Work out the finished part from the listing and answer in its coordinate system (mm). Round coordinates to 2 decimals unless told otherwise and drop trailing zeros. Loops run counter-clockwise (first coordinate to the right, second up) from the corner with the lowest first, then second, coordinate; pieces in that order, holes last.
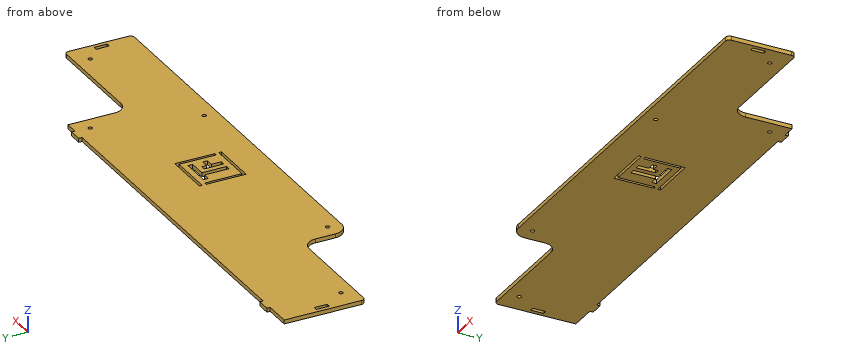
from build123d import *

# Parameters (mm, degrees)
SKETCH001002018_R = 1.5
SKETCH001002018_W = 9.8
SKETCH001002018_H = 3
PAD020_DEPTH      = 3
FILLET031_R       = 3
FILLET032_R       = 10


with BuildPart() as part:
    # Sketch001002018 → Pad020 (new body)
    with BuildSketch(Plane(origin=(0, 45, 17.5), x_dir=(0, -1, 0), z_dir=(0, 0, 1))):
        Polygon((-61, -198.5), (0, -198.5), (0, -108.5), (35, -108.5), (35, 198.5), (-16, 198.5), (-16, 108.5), (-61, 108.5), (-61, 98.5), (-63.5, 98.5), (-63.5, 88.5), (-61, 88.5), (-61, -168.5), (-63.5, -168.5), (-63.5, -178.5), (-61, -178.5), align=None)
        with Locations((-50.1, 97.5)):
            Circle(SKETCH001002018_R, mode=Mode.SUBTRACT)
        with Locations((-5.1, 182.5)):
            Circle(SKETCH001002018_R, mode=Mode.SUBTRACT)
        with Locations((24.9, 77.5)):
            Circle(SKETCH001002018_R, mode=Mode.SUBTRACT)
        with Locations((-10.1, -182.5)):
            Circle(SKETCH001002018_R, mode=Mode.SUBTRACT)
        with Locations((24.9, -97.5)):
            Circle(SKETCH001002018_R, mode=Mode.SUBTRACT)
        with Locations((-30.5, -194)):
            Rectangle(SKETCH001002018_W, SKETCH001002018_H, mode=Mode.SUBTRACT)
        with Locations((9.5, 194)):
            Rectangle(SKETCH001002018_W, SKETCH001002018_H, mode=Mode.SUBTRACT)
        Polygon((-18.6, -7.5), (-18.6, -5.5), (9.4, -5.5), (9.4, 27.5), (11.4, 27.5), (11.4, -7.5), align=None, mode=Mode.SUBTRACT)
        Polygon((-21.6, -7.5), (-23.6, -7.5), (-23.6, 27.5), (6.4, 27.5), (6.4, 25.5), (-21.6, 25.5), align=None, mode=Mode.SUBTRACT)
        Polygon((-13.6, -1), (-17.1, -1), (-17.1, 21), (-13.6, 21), (-13.6, 8), (4.9, 8), (4.9, 4.5), (-13.6, 4.5), align=None, mode=Mode.SUBTRACT)
        Polygon((-9.6, 12), (4.9, 12), (4.9, 15.5), (-2.6, 15.5), (-2.6, 21), (-6.1, 21), (-6.1, 15.5), (-9.6, 15.5), align=None, mode=Mode.SUBTRACT)
    extrude(amount=PAD020_DEPTH)

    # Fillet031
    fillet031_edges = [part.edges().sort_by_distance(p)[0] for p in [
        (-198.5, 45, 19),
        (198.5, 10, 19),
        (198.5, 61, 19),
    ]]
    fillet(fillet031_edges, radius=FILLET031_R)

    # Fillet032
    fillet032_edges = [part.edges().sort_by_distance(p)[0] for p in [
        (-108.5, 45, 19),
        (-108.5, 10, 19),
        (108.5, 61, 19),
    ]]
    fillet(fillet032_edges, radius=FILLET032_R)


solid = part.part
Item 1: Section A-A, the plane z = 19.4 is taken. State how many separate pieces and enclosed holes the cut face has, plus the area to 3 significant figures.
Item 2: Straight lines are drawn through the part: line 1 (Y direction, x = 12.5, z = 17.85); line 2 (X direction, y = 20.1, z = 19.5); line 3 (X direction, y = 80, z = 19.7). For each, find the intervals that lie inside material, in ascending order.
Item 3: Section C-C, the plane x = 134.5 is taken. Give the vertices of the cut face in (y, z), plus the area to 3 significant figures.
Item 4: Each of these flat-tipped pins is pushed along its axis until it touches: P1, Ø1.5, axis at x = 11.5, z = 19, coming from the +Y side; P2, Ø1.5, axis at x = 194.5, z = 18.5, coming from the +Y side; P3, Ø1.5, axis at y = 34, z = 19.5, coming from the -X side. Where does it stop, or does it pass through?
Item 5: Section B-B, the plane x = 58.5 is taken. Give the vertices of the cut face in (y, z), plus the area to 3 significant figures.
Answer below:
1. separate pieces: 1
1. enclosed holes: 11
1. area: 30,400 mm2
2. line 1: y = 10 to 33.6, 35.6 to 40.1, 54.6 to 58.6, 62.1 to 66.6, 68.6 to 106
2. line 2: x = -108.5 to -99, -96 to 76, 79 to 198.5
2. line 3: x = -198.5 to -195.5, -192.5 to 108.5
3. outline: (10, 17.5) - (61, 17.5) - (61, 20.5) - (10, 20.5) - close
3. area: 153 mm2
4. P1: stops at y = 106
4. P2: stops at y = 61
4. P3: stops at x = -108.5
5. outline: (10, 17.5) - (106, 17.5) - (106, 20.5) - (10, 20.5) - close
5. area: 288 mm2
